from build123d import *

# Parameters (mm, degrees)
SKETCH2_W           = 144
SKETCH2_H           = 186
BOSS_EXTRUDE1_DEPTH = 4
SKETCH3_W           = 144
SKETCH3_H           = 186
SKETCH3_W_2         = 136
SKETCH3_H_2         = 178
BOSS_EXTRUDE2_DEPTH = 236.6
SKETCH4_R           = 47.5
CUT_EXTRUDE1_DEPTH  = 4
SKETCH5_R           = 21.65
CUT_EXTRUDE2_DEPTH  = 4
BOSS_EXTRUDE3_START = 103.7
SKETCH6_R           = 25.65
SKETCH6_R_2         = 21.65
BOSS_EXTRUDE3_DEPTH = 103.7


with BuildPart() as part:
    # Sketch2 → Boss-Extrude1 (new body)
    with BuildSketch(Plane(origin=(0, 0, 0), x_dir=(1, 0, 0), z_dir=(0, 1, 0))):
        with Locations((72, 93)):
            Rectangle(SKETCH2_W, SKETCH2_H)
    extrude(amount=BOSS_EXTRUDE1_DEPTH)

    # Sketch3 → Boss-Extrude2 (add)
    with BuildSketch(Plane(origin=(0, 0, 0), x_dir=(-1, 0, 0), z_dir=(0, -1, 0))):
        with Locations((-72, 93)):
            Rectangle(SKETCH3_W, SKETCH3_H)
        with Locations((-72, 93)):
            Rectangle(SKETCH3_W_2, SKETCH3_H_2, mode=Mode.SUBTRACT)
    extrude(amount=BOSS_EXTRUDE2_DEPTH)

    # Sketch4 → Cut-Extrude1 (cut)
    with BuildSketch(Plane(origin=(0, 4, 0), x_dir=(1, 0, 0), z_dir=(0, 1, 0))):
        with Locations(Location((72, 64, 0), (0, 0, 270))):
            Circle(SKETCH4_R)
    extrude(amount=-CUT_EXTRUDE1_DEPTH, mode=Mode.SUBTRACT)

    # Sketch5 → Cut-Extrude2 (cut)
    with BuildSketch(Plane(origin=(0, 0, 0), x_dir=(-1, 0, 0), z_dir=(0, -1, 0))):
        with Locations(Location((-72, 150, 0), (0, 0, 90))):
            Circle(SKETCH5_R)
    extrude(amount=-CUT_EXTRUDE2_DEPTH, mode=Mode.SUBTRACT)

    # Sketch6 → Boss-Extrude3 (add)
    with BuildSketch(Plane(origin=(0, 0, 0), x_dir=(-1, 0, 0), z_dir=(0, -1, 0)).offset(BOSS_EXTRUDE3_START)):
        with Locations(Location((-72, 150, 0), (0, 0, 270))):
            Circle(SKETCH6_R)
        with Locations(Location((-72, 150, 0), (0, 0, 90))):
            Circle(SKETCH6_R_2, mode=Mode.SUBTRACT)
    extrude(amount=-BOSS_EXTRUDE3_DEPTH)


solid = part.part
Work out the finished part from the listing and answer in its coordinate system (mm). A direction names the side the tool comes from. Coordinates: 2 decimals unless noted, no trailing zeros. Order: outer loops, then holes, each group sorted by start corner. A loop starts at its lowest first (then second) coordinate and runs counter-clockwise, first axis right, second up. Notation, with made-up numbers: (62, 60.5) - (114, 60.5) arc R22 cw to (114, 71.5) - close; hole circle Ø8 at (-36, 61). An arc over 180 degrees is marked (long way). Put each result on its own line as item: value. Start each with the question number.
1) Find section D-D (y = -193.5). Give the vertices of the cut face in (x, z).
2) Find the intervals of material crossed by line 1 (X direction, y = -47, z = -150); line 2 (Z direction, x = 31, y = -45); line 3 (X direction, y = 3, z = -64), in increasing order. Write a range as from..to.
3) Find section A-A (y = -18). Give the vertices of the cut face in (x, z), plus the area to 3 significant figures.
4) For a pull along X with two mould halves and no side action, classify faces 3 (the cylindrical face through (64.295, -52.576, -125.534)), 4 (the flat face through (144, -115, -92)), 5 (the flat face through (71, 4, -115)) as released by +X, released by -X, zero draft, split by the parting line, or undercut.
5) For faces 1 (the flat face through (142, -236.6, -93)), 2 (the flat face through (4, -117, -92)), determine the directions among +Z, -Z, +X, -X, +Y, -Y from which every point of the face is accessible in a straight line to the end or side of a thin tool.
6) Find section B-B (z = -64). Give the vertices of the cut face in (x, y).
7) Find section C-C (x = 72). Give the vertices of the cut face in (y, z).
Results list:
1. outline: (0, -186) - (144, -186) - (144, 0) - (0, 0) - close; hole (4, -182) - (140, -182) - (140, -4) - (4, -4) - close
2. line 1: x = 0..4, 46.35..50.35, 93.65..97.65, 140..144
2. line 2: z = -186..-182, -4..0
2. line 3: x = 0..24.5, 119.5..144
3. outline: (0, -186) - (144, -186) - (144, 0) - (0, 0) - close; circle Ø51.3 at (72, -150); hole (4, -182) - (140, -182) - (140, -4) - (4, -4) - close; hole circle Ø43.3 at (72, -150)
3. area: 3,170 mm^2
4. face 3: undercut
4. face 4: released by +X
4. face 5: zero draft
5. face 1: +Z, -Z, +X, -X, -Y
5. face 2: -Y
6. outline: (0, -236.6) - (4, -236.6) - (4, 0) - (24.5, 0) - (24.5, 4) - (0, 4) - close; (119.5, 0) - (140, 0) - (140, -236.6) - (144, -236.6) - (144, 4) - (119.5, 4) - close
7. outline: (-236.6, -186) - (4, -186) - (4, -171.65) - (-103.7, -171.65) - (-103.7, -175.65) - (0, -175.65) - (0, -182) - (-236.6, -182) - close; (-236.6, -4) - (0, -4) - (0, -16.5) - (4, -16.5) - (4, 0) - (-236.6, 0) - close; (-103.7, -128.35) - (4, -128.35) - (4, -111.5) - (0, -111.5) - (0, -124.35) - (-103.7, -124.35) - close
